The model under review builds one solid part; all positions refer to its coordinate system, in mm. A direction names the side the tool comes from. Round coordinates to 2 decimals unless told otherwise and drop trailing zeros. Order: outer loops, then holes, each group sorted by start corner. A loop starts at its lowest first (then second) coordinate and runs counter-clockwise, first axis right, second up. Notation, with made-up numbers: M -18,13.25 L 3,13.25 A21 cw 3,41.25 Z; hole C 57,-32.75 d4. An arc over 180 degrees is marked long. Use a Markdown table: item, result. Add a question column.
1. Consider section A-A on z = 0. State the section outline as (x, y) points.
2. The part is to be moulded in two halves that separate along X. For faces 1 (the flat face through (0, 0, 0)), 2 (the cylindrical face through (-17.319, -3.55, -3.807)), 3 (the flat face through (0, 1.5, -8)), say which applies: +X half, -X half, draft (parallel to the pull), parting line (faces both ways), or undercut.
3. Consider section B-B on y = -3. State the section outline as (x, z) points, then the cut area to 3 significant figures.
4. Insertion check: P1, Ø3, axis at y = -4, z = 3.5, coming from the -X side; P2, Ø3, axis at x = 0, z = 7.58, coming from the -Y side; P3, Ø1.3, axis at x = 9.5, z = -12, coming from the +Y side; P4, Ø1.8, axis at x = -10, z = 0, coming from the +Y side. Each pin has a flat end and moves straight along its axis. Give the tip position at first contact, or say it passes through.
5. Consider section C-C on x = 4.5. State the section outline as (y, z) points.
6. For faces 4 (the flat face through (0, 2.5, 13)), 5 (the flat face through (-5, -5.2, 0)), 6 (the flat face through (0, 4, -10.83)), 7 (the flat face through (12, 1.5, -8)), list the 3-axis set-ups (+Z, -Z, +X, -X, +Y, -Y) from which the entire face can be reached by the end or side of a thin tool; tool diameter is ignored.
7. To check wall thickness, follow probe 1 along X at (y, z) = (-1.75, 0.25); probe 2 along Z at (x, y) = (-10, 1.9); probe 3 along Y at (x, z) = (6, 9.25). State the ranges of each line that lie inside material, in increasing order.
8. Consider section D-D on z = -12. State the section outline as (x, y) points.
from build123d import *

# Parameters (mm, degrees)
SKETCH_1_W                           = 40
SKETCH_1_H                           = 30
EXTRUDE_1_DEPTH                      = 2.5
SKETCH_2_R                           = 8.25
EXTRUDE_2_DEPTH                      = 7.2
CUT_EXTRUDE_START                    = -2
SKETCH_3_R                           = 6.25
CUT_EXTRUDE_1_DEPTH                  = 2
EXTRUDE_4_DEPTH                      = 1.2
SKETCH_4_R                           = 1.15
CUT_EXTRUDE_2_DEPTH                  = 3.7
CUT_EXTRUDE_4_DEPTH                  = 4
CHAMFER_1_SIZE                       = 0.2
EXTRUDE_5_DEPTH                      = 40
SKETCH_9_R                           = 2.25
CUT_EXTRUDE_5_DEPTH                  = 2.2
CUT_EXTRUDE_5_DIRECTION_2_REACH      = 28.816
CUT_EXTRUDE_5_DIRECTION_2_END_RADIUS = 5
SKETCH_13_W                          = 40
SKETCH_13_H                          = 5
EXTRUDE_6_DEPTH                      = 3
SKETCH_14_R                          = 1.75
CUT_EXTRUDE_7_DEPTH                  = 4


with BuildPart() as part:
    # Эскиз1 → Бобышка-Вытянуть1 (new body)
    with BuildSketch(Plane(origin=(0, 0, 0), x_dir=(1, 0, 0), z_dir=(0, 1, 0))):
        Rectangle(SKETCH_1_W, SKETCH_1_H)
    extrude(amount=EXTRUDE_1_DEPTH)

    # Эскиз2 → Бобышка-Вытянуть2 (add)
    with BuildSketch(Plane.XZ):
        with Locations(Location((-10, 0, 0), (0, 0, 270))):
            Circle(SKETCH_2_R)
        with BuildLine():
            Line((-13.1, 5.427015755), (-13.1, -5.427015755))
            ThreePointArc((-13.1, -5.427015755), (-10, -6.25), (-6.9, -5.427015755))
            Line((-6.9, -5.427015755), (-6.9, 5.427015755))
            ThreePointArc((-6.9, 5.427015755), (-10, 6.25), (-13.1, 5.427015755))
        make_face(mode=Mode.SUBTRACT)
    extrude(amount=EXTRUDE_2_DEPTH)

    # Эскиз3 → Вырез-Вытянуть1 (cut)
    with BuildSketch(Plane.XZ.offset(7.2).offset(CUT_EXTRUDE_START)):
        with Locations(Location((-10, 0, 0), (0, 0, 60.264286892))):
            Circle(SKETCH_3_R)
    extrude(amount=CUT_EXTRUDE_1_DEPTH, mode=Mode.SUBTRACT)

    # Эскиз8 → Бобышка-Вытянуть4 (add)
    with BuildSketch(Plane.XZ):
        with BuildLine():
            Line((-13.1, 5.427015755), (-13.1, -5.427015755))
            ThreePointArc((-13.1, -5.427015755), (-10, -6.25), (-6.9, -5.427015755))
            Line((-6.9, -5.427015755), (-6.9, 5.427015755))
            ThreePointArc((-6.9, 5.427015755), (-10, 6.25), (-13.1, 5.427015755))
        make_face()
    extrude(amount=EXTRUDE_4_DEPTH)

    # Эскиз4 → Вырез-Вытянуть2 (cut)
    with BuildSketch(Plane.XZ.offset(-2.5)):
        with Locations(Location((-10, 0, 0), (0, 0, 270))):
            Circle(SKETCH_4_R)
    extrude(amount=CUT_EXTRUDE_2_DEPTH, mode=Mode.SUBTRACT)

    # Эскиз6 → Вырез-Вытянуть4 (cut)
    with BuildSketch(Plane.XZ.offset(5.2)):
        Polygon((-13.1, 1.25), (-13.1, -1.25), (-13.1, -1.45), (-13.682842712, -1.45), (-14.3, -0.832842712), (-14.3, 0.832842712), (-13.682842712, 1.45), (-13.1, 1.45), align=None)
    extrude(amount=-CUT_EXTRUDE_4_DEPTH, mode=Mode.SUBTRACT)

    # Фаска1
    chamfer_1_edges = [part.edges().sort_by_distance(p)[0] for p in [
        (-13.1, -3.2, -1.45),
        (-13.1, -3.2, 1.45),
    ]]
    chamfer(chamfer_1_edges, length=CHAMFER_1_SIZE)

    # Эскиз10 → Бобышка-Вытянуть5 (add)
    with BuildSketch(Plane.ZY.offset(20)):
        with BuildLine():
            Line((-5.830127019, 5.5), (-5.830127019, 2.5))
            Line((-5.830127019, 2.5), (5.830127019, 2.5))
            Line((5.830127019, 2.5), (5.830127019, 5.5))
            Line((5.830127019, 5.5), (4.330127019, 5.5))
            ThreePointArc((4.330127019, 5.5), (0, 3), (-4.330127019, 5.5))
            Line((-4.330127019, 5.5), (-5.830127019, 5.5))
        make_face()
    extrude(amount=-EXTRUDE_5_DEPTH)

    # Эскиз9 → Вырез-Вытянуть5 (cut)
    with BuildSketch(Plane(origin=(0, 2.5, 0), x_dir=(1, 0, 0), z_dir=(0, 1, 0))):
        with Locations(Location((-10, 0, 0), (0, 0, 90))):
            Circle(SKETCH_9_R)
    extrude(amount=-CUT_EXTRUDE_5_DEPTH, mode=Mode.SUBTRACT)

    # Вырез-Вытянуть5 direction 2: up to this cylinder (the profile starts outside it)
    cut_extrude_5_direction_2_end = Plane(origin=(-10, 8, 0), z_dir=(-1, 0, 0)) * Cylinder(CUT_EXTRUDE_5_DIRECTION_2_END_RADIUS, 68.632, mode=Mode.PRIVATE)
    # Эскиз9 → Вырез-Вытянуть5 direction 2 (cut, up to the surface)
    with BuildSketch(Plane(origin=(0, 2.5, 0), x_dir=(1, 0, 0), z_dir=(0, 1, 0)), mode=Mode.PRIVATE) as cut_extrude_5_direction_2_sk1:
        with Locations(Location((-10, 0, 0), (0, 0, 90))):
            Circle(SKETCH_9_R)
    cut_extrude_5_direction_2_tool1 = extrude(cut_extrude_5_direction_2_sk1.sketch, amount=CUT_EXTRUDE_5_DIRECTION_2_REACH, mode=Mode.PRIVATE) - cut_extrude_5_direction_2_end
    add(cut_extrude_5_direction_2_tool1.solids().sort_by_distance((-10, 2.5, 0))[0], mode=Mode.SUBTRACT)

    # Эскиз13 → Бобышка-Вытянуть6 (add)
    with BuildSketch(Plane(origin=(0, 2.5, 0), x_dir=(1, 0, 0), z_dir=(0, 1, 0))):
        with Locations((0, 8.330127019)):
            Rectangle(SKETCH_13_W, SKETCH_13_H)
        with Locations((0, -8.330127019)):
            Rectangle(SKETCH_13_W, SKETCH_13_H)
    extrude(amount=EXTRUDE_6_DEPTH)

    # Эскиз14 → Вырез-Вытянуть7 (cut)
    with BuildSketch(Plane(origin=(0, 5.5, 0), x_dir=(1, 0, 0), z_dir=(0, 1, 0))):
        with Locations(Location((-12.5, 7.580127019, 0), (0, 0, 270))):
            Circle(SKETCH_14_R)
        with Locations(Location((12.5, 7.580127019, 0), (0, 0, 90))):
            Circle(SKETCH_14_R)
        with Locations(Location((0, 7.580127019, 0), (0, 0, 270))):
            Circle(SKETCH_14_R)
        with Locations(Location((12.5, -7.580127019, 0), (0, 0, 270))):
            Circle(SKETCH_14_R)
        with Locations(Location((0, -7.580127019, 0), (0, 0, 90))):
            Circle(SKETCH_14_R)
        with Locations(Location((-12.5, -7.580127019, 0), (0, 0, 90))):
            Circle(SKETCH_14_R)
    extrude(amount=-CUT_EXTRUDE_7_DEPTH, mode=Mode.SUBTRACT)


solid = part.part
Answer block:
| question | item | result |
|---|---|---|
| 1 | outline | M -20,0 L -18.25,0 L -18.25,-7.2 L -16.25,-7.2 L -16.25,-5.2 L -14.3,-5.2 L -14.3,-1.2 L -11.15,-1.2 L -11.15,0.3 L -12.25,0.3 L -12.25,3 L -20,3 Z; M -8.85,-1.2 L -6.9,-1.2 L -6.9,-5.2 L -3.75,-5.2 L -3.75,-7.2 L -1.75,-7.2 L -1.75,0 L 20,0 L 20,3 L -7.75,3 L -7.75,0.3 L -8.85,0.3 Z |
| 2 | face 1 | draft |
| 2 | face 2 | parting line |
| 2 | face 3 | undercut |
| 3 | outline | C -10,0 d16.5; hole M -14.3,-0.83 L -13.68,-1.45 L -13.3,-1.45 L -13.1,-1.65 L -13.1,-5.43 A6.25 ccw -6.9,-5.43 L -6.9,5.43 A6.25 ccw -13.1,5.43 L -13.1,1.65 L -13.3,1.45 L -13.68,1.45 L -14.3,0.83 Z |
| 3 | area | 136 mm^2 |
| 4 | P1 | x = -18 |
| 4 | P2 | y = 0 |
| 4 | P3 | y = 2.5 |
| 4 | P4 | through |
| 5 | outline | M 0,-15 L 2.5,-15 L 2.5,-10.83 L 5.5,-10.83 L 5.5,-4.33 A5 cw 5.5,4.33 L 5.5,10.83 L 2.5,10.83 L 2.5,15 L 0,15 Z |
| 6 | face 4 | +Z, +X, -X, +Y |
| 6 | face 5 | -Y |
| 6 | face 6 | -Z, +X, -X, +Y |
| 6 | face 7 | +Y |
| 7 | probe 1 | -18.25 to -14.3, -6.9 to -1.75 |
| 7 | probe 2 | -15 to -2.25, 2.25 to 15 |
| 7 | probe 3 | 0 to 5.5 |
| 8 | outline | M -20,0 L 20,0 L 20,2.5 L -20,2.5 Z |
